```python
from build123d import *

# Parameters (mm, degrees)
CYLINDER011_R     = 4
CYLINDER011_DEPTH = 28.5
CYLINDER007_R     = 2.25
CYLINDER007_DEPTH = 65
CYLINDER006_R     = 2.25
CYLINDER006_DEPTH = 65
PAD002_DEPTH      = 4
PAD001_DEPTH      = 4
CYLINDER010_R     = 4
CYLINDER010_DEPTH = 28.5
CYLINDER004_R     = 2.25
CYLINDER004_DEPTH = 10
CYLINDER005_R     = 4
CYLINDER005_DEPTH = 5
CYLINDER002_R     = 2.25
CYLINDER002_DEPTH = 10
CYLINDER003_R     = 4
CYLINDER003_DEPTH = 5
CYLINDER_R        = 22.5
CYLINDER_DEPTH    = 10
BOX_W             = 100
BOX_H             = 10
BOX_DEPTH         = 10
BOX001_W          = 65
BOX001_H          = 10
BOX001_DEPTH      = 37.5
FILLET_R          = 2


with BuildPart() as cylinder011:
    # Cylinder011 → Cylinder011 (new body)
    with BuildSketch(Plane(origin=(-27.5, 5, 0), x_dir=(1, 0, 0), z_dir=(0, 0, 1))):
        Circle(CYLINDER011_R)
    extrude(amount=CYLINDER011_DEPTH)


with BuildPart() as cylinder007:
    # Cylinder007 → Cylinder007 (new body)
    with BuildSketch(Plane(origin=(-27.5, 5, 0), x_dir=(1, 0, 0), z_dir=(0, 0, 1))):
        Circle(CYLINDER007_R)
    extrude(amount=CYLINDER007_DEPTH)


with BuildPart() as fusion004:
    # Cylinder006 → Cylinder006 (new body)
    with BuildSketch(Plane(origin=(27.5, 5, 0), x_dir=(1, 0, 0), z_dir=(0, 0, 1))):
        Circle(CYLINDER006_R)
    extrude(amount=CYLINDER006_DEPTH)

    # Fusion004: union Cylinder007
    add(cylinder007.part)


with BuildPart() as m4press001:
    # Sketch002 → Pad002 (new body)
    with BuildSketch(Plane.XY):
        Polygon((4, 0), (2, 3.464102), (-2, 3.464102), (-4, 0), (-2, -3.464102), (2, -3.464102), align=None)
    extrude(amount=PAD002_DEPTH)


with BuildPart() as m4press001_1:
    # Body002 placement: moved
    add(m4press001.part.moved(Location((27.5, 5, 28.5))))


with BuildPart() as m4press:
    # Sketch001 → Pad001 (new body)
    with BuildSketch(Plane.XY):
        Polygon((4, 0), (2, 3.464102), (-2, 3.464102), (-4, 0), (-2, -3.464102), (2, -3.464102), align=None)
    extrude(amount=PAD001_DEPTH)


with BuildPart() as m4press_1:
    # Body001 placement: moved
    add(m4press.part.moved(Location((-27.5, 5, 28.5))))


with BuildPart() as connectors:
    # Cylinder010 → Cylinder010 (new body)
    with BuildSketch(Plane(origin=(27.5, 5, 0), x_dir=(1, 0, 0), z_dir=(0, 0, 1))):
        Circle(CYLINDER010_R)
    extrude(amount=CYLINDER010_DEPTH)

    # Fusion006: union Cylinder011, Fusion004, M4Press001, M4Press
    add(cylinder011.part)
    add(fusion004.part)
    add(m4press001_1.part)
    add(m4press_1.part)


with BuildPart() as cylinder004:
    # Cylinder004 → Cylinder004 (new body)
    with BuildSketch(Plane.XY):
        Circle(CYLINDER004_R)
    extrude(amount=CYLINDER004_DEPTH)


with BuildPart() as fusion002:
    # Cylinder005 → Cylinder005 (new body)
    with BuildSketch(Plane.XY.offset(5)):
        Circle(CYLINDER005_R)
    extrude(amount=CYLINDER005_DEPTH)

    # Fusion002: union Cylinder004
    add(cylinder004.part)


with BuildPart() as fusion002_1:
    # Fusion002 placement: moved
    add(fusion002.part.moved(Location((-40, 5, 0))))


with BuildPart() as cylinder002:
    # Cylinder002 → Cylinder002 (new body)
    with BuildSketch(Plane.XY):
        Circle(CYLINDER002_R)
    extrude(amount=CYLINDER002_DEPTH)


with BuildPart() as fusion003:
    # Cylinder003 → Cylinder003 (new body)
    with BuildSketch(Plane.XY.offset(5)):
        Circle(CYLINDER003_R)
    extrude(amount=CYLINDER003_DEPTH)

    # Fusion001: union Cylinder002
    add(cylinder002.part)


with BuildPart() as fusion003_1:
    # Fusion001 placement: moved
    add(fusion003.part.moved(Location((40, 5, 0))))

    # Fusion003: union Fusion002
    add(fusion002_1.part)


with BuildPart() as cylinder:
    # Cylinder → Cylinder (new body)
    with BuildSketch(Plane(origin=(0, 10, 37.5), x_dir=(1, 0, 0), z_dir=(0, -1, 0))):
        Circle(CYLINDER_R)
    extrude(amount=CYLINDER_DEPTH)


with BuildPart() as cube:
    # Box → Box (new body)
    with BuildSketch(Plane(origin=(-50, 0, 0), x_dir=(1, 0, 0), z_dir=(0, 0, 1))):
        with Locations((50, 5)):
            Rectangle(BOX_W, BOX_H)
    extrude(amount=BOX_DEPTH)


with BuildPart() as lower_part:
    # Box001 → Box001 (new body)
    with BuildSketch(Plane(origin=(-32.5, 0, 0), x_dir=(1, 0, 0), z_dir=(0, 0, 1))):
        with Locations((32.5, 5)):
            Rectangle(BOX001_W, BOX001_H)
    extrude(amount=BOX001_DEPTH)

    # Fusion: union Cube
    add(cube.part)

    # Cut: cut Cylinder
    add(cylinder.part, mode=Mode.SUBTRACT)

    # Cut001: cut Fusion003
    add(fusion003_1.part, mode=Mode.SUBTRACT)

    # Cut002: cut Connectors
    add(connectors.part, mode=Mode.SUBTRACT)

    # Fillet
    fillet_edges = [lower_part.edges().sort_by_distance(p)[0] for p in [
        (50, 5, 10),
        (32.5, 5, 10),
        (32.5, 5, 37.5),
        (22.5, 5, 37.5),
        (-22.5, 5, 37.5),
        (-32.5, 5, 37.5),
        (-32.5, 5, 10),
        (-50, 5, 10),
    ]]
    fillet(fillet_edges, radius=FILLET_R)


solid = lower_part.part
```
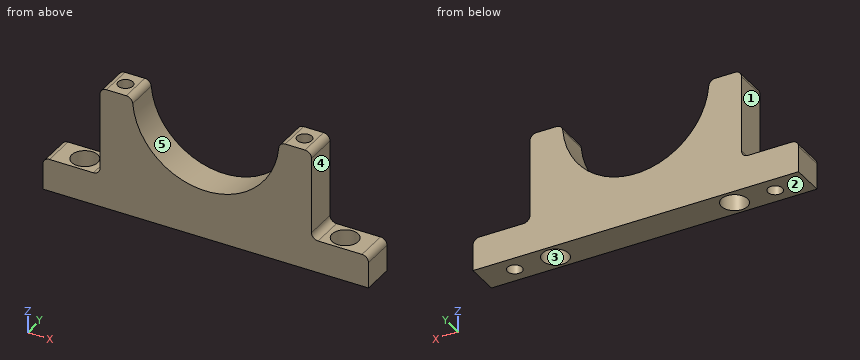
The model under review builds one solid part; all positions refer to its coordinate system, in mm. Face numbers are marked on the shaded views. A direction names the side the tool comes from. Round coordinates to 2 decimals unless told otherwise and drop trailing zeros. Order: outer loops, then holes, each group sorted by start corner. A loop starts at its lowest first (then second) coordinate and runs counter-clockwise, first axis right, second up.
Item 1: Machinability: for the marked faces 4 and 5, which of the approach directions +Z, -Z, +X, -X, +Y, -Y give a long, thin tool a straight path to every point of the face, cutting with its end or side? Answer none if there is none.
Working result:
face 4: +Z, +X, +Y, -Y
face 5: +Z, +Y, -Y
Item 2: For pin 1 (2 mm diameter, centred on x = -7.5, z = 16.5, fed in from -Y); pin 2 (2 mm diameter, centred on x = -25, y = 6.5, fed in from -Z); pin 3 (4 mm diameter, centred on x = 40.5, y = 3.5, fed in from +Z); pin 4 (6 mm diameter, centred on x = 20, y = 7, fed in from +Z), all flat-tipped, find the tip position at first contact; note any pin that passes through.
Working result:
pin 1: stops at y = 0
pin 2: stops at z = 28.5
pin 3: stops at z = 5
pin 4: stops at z = 36.91
Item 3: Add section D-D, the plane x = 0. State the section outline as (y, z) points, and give its area (3 significant figures).
Working result:
outline: (0, 0) - (10, 0) - (10, 15) - (0, 15) - close
area: 150 mm2
Item 4: Draft analysis for pull direction X (two halves, no side actions). For the marked faces 1, 2 and 3, state which applies: released by +X, released by -X, zero draft, split by the parting line, or undercut.
Working result:
face 1: released by -X
face 2: zero draft
face 3: undercut
Item 5: Add section B-B, the plane z = 21. State the section outline as (x, y) points.
Working result:
outline: (-32.5, 0) - (-15.3, 0) - (-15.3, 10) - (-32.5, 10) - close; (15.3, 0) - (32.5, 0) - (32.5, 10) - (15.3, 10) - close; hole circle Ø8 at (-27.5, 5); hole circle Ø8 at (27.5, 5)
Item 6: Add section A-A, the plane x = 40. State the section outline as (y, z) points.
Working result:
outline: (0, 0) - (2.75, 0) - (2.75, 5) - (1, 5) - (1, 10) - (0, 10) - close; (7.25, 0) - (10, 0) - (10, 10) - (9, 10) - (9, 5) - (7.25, 5) - close
Item 7: Add section C-C, the plane x = 27.5. State the section outline as (y, z) points.
Working result:
outline: (0, 0) - (1, 0) - (1, 28.5) - (1.54, 28.5) - (1.54, 32.5) - (2.75, 32.5) - (2.75, 37.5) - (0, 37.5) - close; (7.25, 32.5) - (8.46, 32.5) - (8.46, 28.5) - (9, 28.5) - (9, 0) - (10, 0) - (10, 37.5) - (7.25, 37.5) - close
Item 8: To check wall thickness, follow probe 1 along Y at (x, z) = (27.5, 15); probe 2 along X at (y, z) = (5, 34.55); probe 3 along X at (y, z) = (3, 19.5). State the ranges of each line that lie inside material, in increasing order.
Working result:
probe 1: y = 0 to 1, 9 to 10
probe 2: x = -32.5 to -29.75, -25.25 to -22.31, 22.31 to 25.25, 29.75 to 32.5
probe 3: x = -32.5 to -30.96, -24.04 to -13.5, 13.5 to 24.04, 30.96 to 32.5
